For this review, take the finished solid that the model builds, in its own axes (mm). A direction names the side the tool comes from. Coordinates: 2 decimals unless noted, no trailing zeros. Write each loop counter-clockwise with the first axis right and the second up, starting at its lowest first coordinate (ties: lowest second). Pieces come first, ordered by that corner, then holes. Notation, with made-up numbers: M -27,62 L -16,62 A22 ccw -16,75 Z; hole C 45.5,37 d1. An arc over 180 degrees is marked long. One line per question, with ' | ' between items.
from build123d import *

# Parameters (mm, degrees)
SKETCH_1_R            = 18.575
GEAR_BOX_DEPTH        = 22.8
SKETCH_1_3_R          = 17.35
MOTOR_DEPTH           = 65
SKETCH_2_R            = 6
SKETCH_2_R_2          = 3
CU_BEARING_DEPTH      = 6
SKETCH_2_3_R          = 3
F_6MMSHAFT_DEPTH      = 31
SKETCH_2_4_R          = 1
M2_TAPPING_HOLE_DEPTH = 5


with BuildPart() as part:
    # Sketch 1 → gear box (new body)
    with BuildSketch(Plane(origin=(0, 0, 0), x_dir=(1, 0, 0), z_dir=(0, 1, 0))):
        with Locations(Location((0, 0, 0), (0, 0, 270))):
            Circle(SKETCH_1_R)
    extrude(amount=GEAR_BOX_DEPTH)

    # Sketch 1_3 → motor (add)
    with BuildSketch(Plane(origin=(0, 0, 0), x_dir=(1, 0, 0), z_dir=(0, 1, 0))):
        with Locations(Location((0, 0, 0), (0, 0, 270))):
            Circle(SKETCH_1_3_R)
    extrude(amount=MOTOR_DEPTH)

    # Sketch 2 → Cu bearing (add)
    with BuildSketch(Plane.XZ):
        with Locations(Location((0, 6.5, 0), (0, 0, 90))):
            Circle(SKETCH_2_R)
        with Locations(Location((0, 6.5, 0), (0, 0, 270))):
            Circle(SKETCH_2_R_2, mode=Mode.SUBTRACT)
    extrude(amount=CU_BEARING_DEPTH)

    # Sketch 2_3 → 6mmshaft (add)
    with BuildSketch(Plane.XZ):
        with Locations(Location((0, 6.5, 0), (0, 0, 270))):
            Circle(SKETCH_2_3_R)
    extrude(amount=F_6MMSHAFT_DEPTH)

    # Sketch 2_4 → M2 tapping hole (cut)
    with BuildSketch(Plane.XZ):
        with Locations(Location((-14, 0, 0), (0, 0, 270))):
            Circle(SKETCH_2_4_R)
        with Locations(Location((14, 0, 0), (0, 0, 270))):
            Circle(SKETCH_2_4_R)
    extrude(amount=-M2_TAPPING_HOLE_DEPTH, mode=Mode.SUBTRACT)


solid = part.part
1. Take a section at D-D on x = 4. State the section outline as (y, z) points, plus the area to 3 significant figures.
Computed values:
outline: M -6,2.03 L 0,2.03 L 0,-18.14 L 22.8,-18.14 L 22.8,-16.88 L 65,-16.88 L 65,16.88 L 22.8,16.88 L 22.8,18.14 L 0,18.14 L 0,10.97 L -6,10.97 Z | area: 2,310 mm2
2. Machinability: for faces 4 (the flat face through (0, 65, 0)), 5 (the flat face through (14, 5, 0)), 6 (the flat face through (17, 22.8, -6)), which of the approach directions +Z, -Z, +X, -X, +Y, -Y give a long, thin tool a straight path to every point of the face, cutting with its end or side? Answer none if there is none.
Computed values:
face 4: +Z, -Z, +X, -X, +Y | face 5: -Y | face 6: +Y
3. Take a section at C-C on y = 43.5. State the section outline as (x, z) points.
Computed values:
outline: C 0,0 d34.7
4. Take a section at B-B on z = 14. State the section outline as (x, y) points, plus the area to 3 significant figures.
Computed values:
outline: M -12.21,0 L 12.21,0 L 12.21,22.8 L 10.25,22.8 L 10.25,65 L -10.25,65 L -10.25,22.8 L -12.21,22.8 Z | area: 1,420 mm2
5. Take a section at A-A on x = 0. State the section outline as (y, z) points (3 decimals), plus the area to 3 significant figures.
Computed values:
outline: M -31,3.5 L -6,3.5 L -6,0.5 L 0,0.5 L 0,-18.575 L 22.8,-18.575 L 22.8,-17.35 L 65,-17.35 L 65,17.35 L 22.8,17.35 L 22.8,18.575 L 0,18.575 L 0,12.5 L -6,12.5 L -6,9.5 L -31,9.5 Z | area: 2,530 mm2
6. Clearance check with flat-ended pins moving along their axes: P1, Ø2, axis at x = 14, z = -0.5, coming from the -Y side; P2, Ø1.6, axis at x = -14, z = 0, coming from the -Y side; P3, Ø1.5, axis at y = 35.5, z = -1, coming from the -X side; P4, Ø18.5, axis at x = -3.5, z = 6.5, coming from the -Y side. State where each tip first meets the part, or that it passes through.
Computed values:
P1: stops at y = 0 | P2: stops at y = 5 | P3: stops at x = -17.35 | P4: stops at y = -31
7. Draft analysis for pull direction Z (two halves, no side actions). For faces 1 (the cylindrical face through (0.9, -18.32, 3.64)), 2 (the flat face through (0, 0, 0)), 3 (the cylindrical face through (13, 2, 0)), state which applies: pulls with the +Z half, pulls with the -Z half, needs draft (parallel to the pull), parting line crosses it, or undercut.
Computed values:
face 1: parting line crosses it | face 2: needs draft | face 3: undercut
8. For line 1 along X through (y, z) = (3, 0) (3 decimals); line 2 along X through (y, z) = (3.5, -0.5); line 3 along Y through (x, z) = (-3, 4), list the stretches that pass through material, from the lowest coordinate up.
Computed values:
line 1: x = -18.575 to -15, -13 to 13, 15 to 18.575 | line 2: x = -18.57 to -14.87, -13.13 to 13.13, 14.87 to 18.57 | line 3: y = -6 to 65
